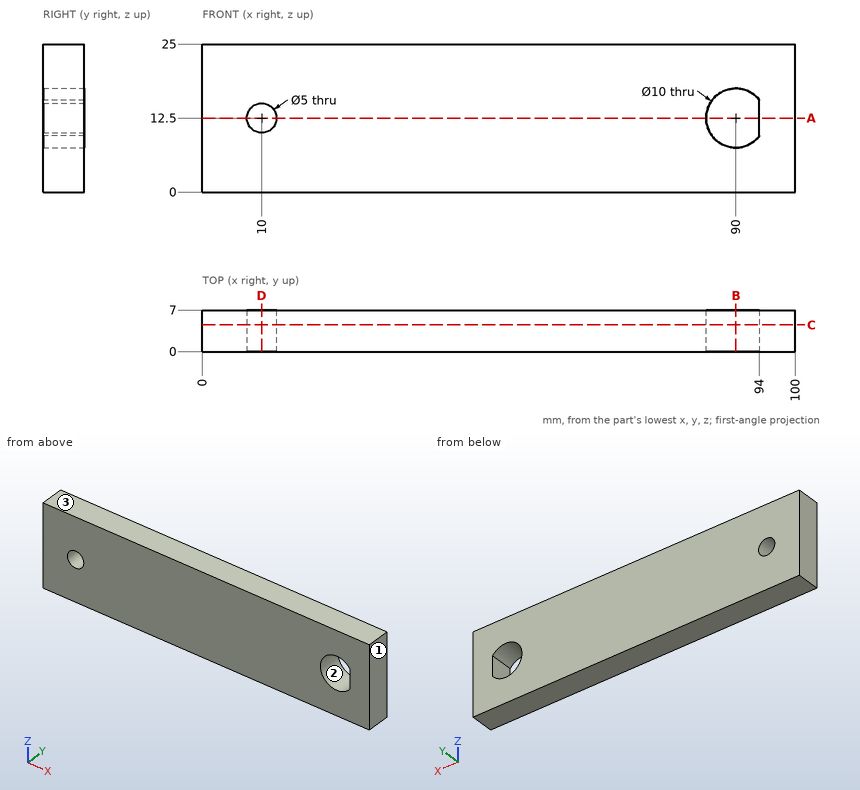
Print and shaded views of the part. All mm, measured from the part's lowest x, y and z. Coordinates: 2 decimals unless noted, no trailing zeros. Order: outer loops, then holes, each group sorted by start corner. A loop starts at its lowest first (then second) coordinate and runs counter-clockwise, first axis right, second up.
(1) Pull direction X, two halves, no side cores. Call the marked faces 1, 2 and 3: pulls with the +X half, pulls with the -X half, needs draft (parallel to the pull), parting line crosses it, or undercut.
Check sheet entries:
face 1: pulls with the +X half
face 2: undercut
face 3: needs draft
(2) Slice it at C-C, the plane y = 4.5. Write the cut outline in (x, z), and give its area (3 significant figures).
Check sheet entries:
outline: (0, 0) - (100, 0) - (100, 25) - (0, 25) - close; hole circle Ø5 at (10, 12.5); hole (94, 9.5) - (94, 15.5) arc R5 ccw (long way) to start
area: 2,410 mm2
(3) Slice it at A-A, the plane z = 12.5. Write the cut outline in (x, y).
Check sheet entries:
outline: (0, 0) - (7.5, 0) - (7.5, 7) - (0, 7) - close; (12.5, 0) - (85, 0) - (85, 7) - (12.5, 7) - close; (94, 0) - (100, 0) - (100, 7) - (94, 7) - close
(4) Slice it at B-B, the plane x = 90. Write the cut outline in (y, z).
Check sheet entries:
outline: (0, 0) - (7, 0) - (7, 7.5) - (0, 7.5) - close; (0, 17.5) - (7, 17.5) - (7, 25) - (0, 25) - close
(5) Slice it at D-D, the plane x = 10. Write the cut outline in (y, z).
Check sheet entries:
outline: (0, 0) - (7, 0) - (7, 10) - (0, 10) - close; (0, 15) - (7, 15) - (7, 25) - (0, 25) - close
(6) Probe L1, parallel to Z at x = 10, y = 2; L2, parallel to Z at x = 90, y = 1.5; L3, parallel to X at y = 6.5, z = 14.25. List the from-to ranges inside material, lowest first.
Check sheet entries:
L1: z = 0 to 10, 15 to 25
L2: z = 0 to 7.5, 17.5 to 25
L3: x = 0 to 8.21, 11.79 to 85.32, 94 to 100
